from build123d import *

# Parameters (mm, degrees)
F0_R     = 3
F0_R_2   = 2
F1_DEPTH = 3
F2_DEPTH = 20
F3_DEPTH = 25
F4_START = 1
F4_DEPTH = 2
F5_SIZE  = 0.2
F6_SIZE  = 0.5


with BuildPart() as f1:
    # F0 (on Top) → F1 (new body)
    with BuildSketch(Plane.XY):
        Circle(F0_R)
        Circle(F0_R_2, mode=Mode.SUBTRACT)
        Circle(F0_R_2)
        Polygon((1.5, 0.8660254038), (1.5, 0), (1.5, -0.8660254038), (0.7499999928, -1.2990381098), (0, -1.7320508076), (-0.7499999928, -1.2990381098), (-1.5, -0.8660254038), (-1.5, 0), (-1.5, 0.8660254038), (-0.7499999928, 1.2990381098), (0, 1.7320508076), (0.7499999928, 1.2990381098), align=None, mode=Mode.SUBTRACT)
        with BuildLine():
            ThreePointArc((0.7499999928, -1.2990381098), (1.2990381036, -0.7500000036), (1.5, 0))
            ThreePointArc((1.5, 0), (1.2990381036, 0.7500000036), (0.7499999928, 1.2990381098))
            ThreePointArc((0.7499999928, 1.2990381098), (0, 1.5), (-0.7499999928, 1.2990381098))
            ThreePointArc((-0.7499999928, 1.2990381098), (-1.2990381036, 0.7500000036), (-1.5, 0))
            ThreePointArc((-1.5, 0), (-1.2990381036, -0.7500000036), (-0.7499999928, -1.2990381098))
            ThreePointArc((-0.7499999928, -1.2990381098), (0, -1.5), (0.7499999928, -1.2990381098))
        make_face()
        with BuildLine():
            Line((0, -1.7320508076), (0.7499999928, -1.2990381098))
            ThreePointArc((0.7499999928, -1.2990381098), (0, -1.5), (-0.7499999928, -1.2990381098))
            Line((-0.7499999928, -1.2990381098), (0, -1.7320508076))
        make_face()
        with BuildLine():
            Line((1.5, -0.8660254038), (1.5, 0))
            ThreePointArc((1.5, 0), (1.2990381036, -0.7500000036), (0.7499999928, -1.2990381098))
            Line((0.7499999928, -1.2990381098), (1.5, -0.8660254038))
        make_face()
        with BuildLine():
            ThreePointArc((0.7499999928, 1.2990381098), (1.2990381036, 0.7500000036), (1.5, 0))
            Line((1.5, 0), (1.5, 0.8660254038))
            Line((1.5, 0.8660254038), (0.7499999928, 1.2990381098))
        make_face()
        with BuildLine():
            ThreePointArc((-0.7499999928, 1.2990381098), (0, 1.5), (0.7499999928, 1.2990381098))
            Line((0.7499999928, 1.2990381098), (0, 1.7320508076))
            Line((0, 1.7320508076), (-0.7499999928, 1.2990381098))
        make_face()
        with BuildLine():
            ThreePointArc((-1.5, 0), (-1.2990381036, 0.7500000036), (-0.7499999928, 1.2990381098))
            Line((-0.7499999928, 1.2990381098), (-1.5, 0.8660254038))
            Line((-1.5, 0.8660254038), (-1.5, 0))
        make_face()
        with BuildLine():
            Line((-1.5, -0.8660254038), (-0.7499999928, -1.2990381098))
            ThreePointArc((-0.7499999928, -1.2990381098), (-1.2990381036, -0.7500000036), (-1.5, 0))
            Line((-1.5, 0), (-1.5, -0.8660254038))
        make_face()
    extrude(amount=F1_DEPTH)

    # F0 (on Top) → F2 (join)
    with BuildSketch(Plane.XY):
        Circle(F0_R_2)
        Polygon((1.5, 0.8660254038), (1.5, 0), (1.5, -0.8660254038), (0.7499999928, -1.2990381098), (0, -1.7320508076), (-0.7499999928, -1.2990381098), (-1.5, -0.8660254038), (-1.5, 0), (-1.5, 0.8660254038), (-0.7499999928, 1.2990381098), (0, 1.7320508076), (0.7499999928, 1.2990381098), align=None, mode=Mode.SUBTRACT)
        with BuildLine():
            ThreePointArc((0.7499999928, -1.2990381098), (1.2990381036, -0.7500000036), (1.5, 0))
            ThreePointArc((1.5, 0), (1.2990381036, 0.7500000036), (0.7499999928, 1.2990381098))
            ThreePointArc((0.7499999928, 1.2990381098), (0, 1.5), (-0.7499999928, 1.2990381098))
            ThreePointArc((-0.7499999928, 1.2990381098), (-1.2990381036, 0.7500000036), (-1.5, 0))
            ThreePointArc((-1.5, 0), (-1.2990381036, -0.7500000036), (-0.7499999928, -1.2990381098))
            ThreePointArc((-0.7499999928, -1.2990381098), (0, -1.5), (0.7499999928, -1.2990381098))
        make_face()
        with BuildLine():
            Line((0, -1.7320508076), (0.7499999928, -1.2990381098))
            ThreePointArc((0.7499999928, -1.2990381098), (0, -1.5), (-0.7499999928, -1.2990381098))
            Line((-0.7499999928, -1.2990381098), (0, -1.7320508076))
        make_face()
        with BuildLine():
            Line((1.5, -0.8660254038), (1.5, 0))
            ThreePointArc((1.5, 0), (1.2990381036, -0.7500000036), (0.7499999928, -1.2990381098))
            Line((0.7499999928, -1.2990381098), (1.5, -0.8660254038))
        make_face()
        with BuildLine():
            ThreePointArc((0.7499999928, 1.2990381098), (1.2990381036, 0.7500000036), (1.5, 0))
            Line((1.5, 0), (1.5, 0.8660254038))
            Line((1.5, 0.8660254038), (0.7499999928, 1.2990381098))
        make_face()
        with BuildLine():
            ThreePointArc((-0.7499999928, 1.2990381098), (0, 1.5), (0.7499999928, 1.2990381098))
            Line((0.7499999928, 1.2990381098), (0, 1.7320508076))
            Line((0, 1.7320508076), (-0.7499999928, 1.2990381098))
        make_face()
        with BuildLine():
            ThreePointArc((-1.5, 0), (-1.2990381036, 0.7500000036), (-0.7499999928, 1.2990381098))
            Line((-0.7499999928, 1.2990381098), (-1.5, 0.8660254038))
            Line((-1.5, 0.8660254038), (-1.5, 0))
        make_face()
        with BuildLine():
            Line((-1.5, -0.8660254038), (-0.7499999928, -1.2990381098))
            ThreePointArc((-0.7499999928, -1.2990381098), (-1.2990381036, -0.7500000036), (-1.5, 0))
            Line((-1.5, 0), (-1.5, -0.8660254038))
        make_face()
    extrude(amount=-F2_DEPTH)

    # F0 (on Top) → F3 (join)
    with BuildSketch(Plane.XY):
        with BuildLine():
            ThreePointArc((0.7499999928, -1.2990381098), (1.2990381036, -0.7500000036), (1.5, 0))
            ThreePointArc((1.5, 0), (1.2990381036, 0.7500000036), (0.7499999928, 1.2990381098))
            ThreePointArc((0.7499999928, 1.2990381098), (0, 1.5), (-0.7499999928, 1.2990381098))
            ThreePointArc((-0.7499999928, 1.2990381098), (-1.2990381036, 0.7500000036), (-1.5, 0))
            ThreePointArc((-1.5, 0), (-1.2990381036, -0.7500000036), (-0.7499999928, -1.2990381098))
            ThreePointArc((-0.7499999928, -1.2990381098), (0, -1.5), (0.7499999928, -1.2990381098))
        make_face()
    extrude(amount=-F3_DEPTH)

    # F0 (on Top) → F4 (cut)
    with BuildSketch(Plane.XY.offset(F4_START)):
        with BuildLine():
            ThreePointArc((0.7499999928, -1.2990381098), (1.2990381036, -0.7500000036), (1.5, 0))
            ThreePointArc((1.5, 0), (1.2990381036, 0.7500000036), (0.7499999928, 1.2990381098))
            ThreePointArc((0.7499999928, 1.2990381098), (0, 1.5), (-0.7499999928, 1.2990381098))
            ThreePointArc((-0.7499999928, 1.2990381098), (-1.2990381036, 0.7500000036), (-1.5, 0))
            ThreePointArc((-1.5, 0), (-1.2990381036, -0.7500000036), (-0.7499999928, -1.2990381098))
            ThreePointArc((-0.7499999928, -1.2990381098), (0, -1.5), (0.7499999928, -1.2990381098))
        make_face()
        with BuildLine():
            ThreePointArc((-0.7499999928, 1.2990381098), (0, 1.5), (0.7499999928, 1.2990381098))
            Line((0.7499999928, 1.2990381098), (0, 1.7320508076))
            Line((0, 1.7320508076), (-0.7499999928, 1.2990381098))
        make_face()
        with BuildLine():
            ThreePointArc((0.7499999928, 1.2990381098), (1.2990381036, 0.7500000036), (1.5, 0))
            Line((1.5, 0), (1.5, 0.8660254038))
            Line((1.5, 0.8660254038), (0.7499999928, 1.2990381098))
        make_face()
        with BuildLine():
            Line((1.5, -0.8660254038), (1.5, 0))
            ThreePointArc((1.5, 0), (1.2990381036, -0.7500000036), (0.7499999928, -1.2990381098))
            Line((0.7499999928, -1.2990381098), (1.5, -0.8660254038))
        make_face()
        with BuildLine():
            Line((0, -1.7320508076), (0.7499999928, -1.2990381098))
            ThreePointArc((0.7499999928, -1.2990381098), (0, -1.5), (-0.7499999928, -1.2990381098))
            Line((-0.7499999928, -1.2990381098), (0, -1.7320508076))
        make_face()
        with BuildLine():
            ThreePointArc((-1.5, 0), (-1.2990381036, 0.7500000036), (-0.7499999928, 1.2990381098))
            Line((-0.7499999928, 1.2990381098), (-1.5, 0.8660254038))
            Line((-1.5, 0.8660254038), (-1.5, 0))
        make_face()
        with BuildLine():
            Line((-1.5, -0.8660254038), (-0.7499999928, -1.2990381098))
            ThreePointArc((-0.7499999928, -1.2990381098), (-1.2990381036, -0.7500000036), (-1.5, 0))
            Line((-1.5, 0), (-1.5, -0.8660254038))
        make_face()
    extrude(amount=F4_DEPTH, mode=Mode.SUBTRACT)

    # F5
    f5_edges = [f1.edges().sort_by_distance(p)[0] for p in [
        (-3, 0, 3),
        (-0.75, 1.299038, 3),
        (0.75, 1.299038, 3),
        (1.5, 0, 3),
        (0.75, -1.299038, 3),
        (-1.5, 0, 3),
        (-0.75, -1.299038, 3),
        (-3, 0, 0),
    ]]
    chamfer(f5_edges, length=F5_SIZE)

    # F6
    f6_edges = [f1.edges().sort_by_distance(p)[0] for p in [
        (0.75, -1.299038, -25),
    ]]
    chamfer(f6_edges, length=F6_SIZE)


solid = f1.part
Geometry: final body of the model. Coordinates: model frame, mm. A direction names the side the tool comes from. Round coordinates to 2 decimals unless told otherwise and drop trailing zeros. Order: outer loops, then holes, each group sorted by start corner. A loop starts at its lowest first (then second) coordinate and runs counter-clockwise, first axis right, second up.
Q1. Section B-B, the plane z = -2.5. Output: boundary loops of the cut face in (x, y), and give its area (3 significant figures).
Result sheet:
outline: circle Ø4 at (0, 0)
area: 12.6 mm2
Q2. Mould query, pull axis Y, two halves, no side actions, for faces 1 (the face through (0, 0, 1)), 2 (the face through (0, -2, -10)), 3 (the face through (-2, 1, 0)). Classes: released by +Y, released by -Y, zero draft, split by the parting line, or undercut.
Result sheet:
face 1: undercut
face 2: split by the parting line
face 3: zero draft
Q3. Section A-A, the plane z = -22.75. Output: boundary loops of the cut face in (x, y), and give its area (3 significant figures).
Result sheet:
outline: circle Ø3 at (0, 0)
area: 7.07 mm2
Q4. Access query for faces 4 (the face through (0, 0, -25)), 5 (the face through (-1.5, 0, 2)). Directions: +Z, -Z, +X, -X, +Y, -Y. A direction counts if a zero-diameter tool reaches every point of the face in a straight line with its end or side. Return the directions, or none.
Result sheet:
face 4: -Z, +X, -X, +Y, -Y
face 5: +Z
Q5. Pin query (flat end, axial travel): pin 1 (2 mm diameter, centred on x = 2, y = -2, fed in from -Z); pin 2 (3 mm diameter, centred on y = 2, z = -1, fed in from -X); pin 3 (1 mm diameter, centred on x = 2, z = -17.5, fed in from +Y). Return the tip coordinate at first contact, or that it passes through.
Result sheet:
pin 1: stops at z = -20
pin 2: stops at x = -2.79
pin 3: stops at y = 1.32
Q6. Material intervals for probe 1 along Z at (x, y) = (0.4, 0.5); probe 2 along X at (y, z) = (2.45, 1.5); probe 3 along Z at (x, y) = (-2.25, 1.1), sorted ascending.
Result sheet:
probe 1: z = -25 to 1
probe 2: x = -1.73 to 1.73
probe 3: z = 0 to 3
